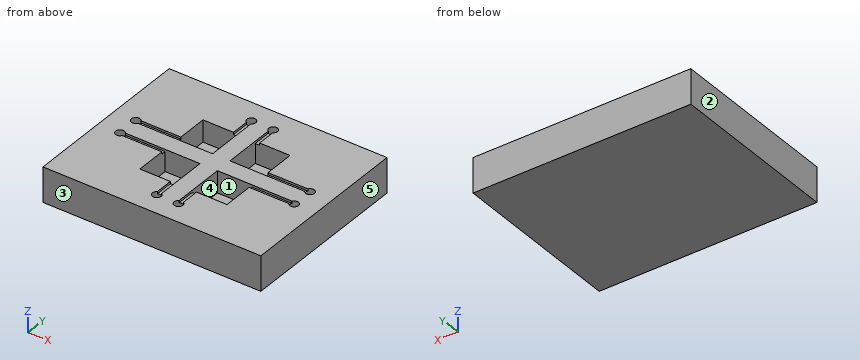
from build123d import *

# Parameters (mm, degrees)
F0_W     = 8
F0_H     = 8
F1_DEPTH = 5
F2_W     = 50
F2_H     = 40
F3_DEPTH = 3
F4_W     = 1
F4_H     = 5
F4_W_2   = 10
F4_H_2   = 1
F5_DEPTH = 0.5
F6_R     = 1
F7_DEPTH = 5


with BuildPart() as f1:
    # F0 (on Top) → F1 (new body)
    with BuildSketch(Plane.XY):
        Polygon((-25, -20), (25, -20), (25, 20), (-10, 20), (-25, 20), align=None)
        with Locations((-6, -6)):
            Rectangle(F0_W, F0_H, mode=Mode.SUBTRACT)
        with Locations((6, -6)):
            Rectangle(F0_W, F0_H, mode=Mode.SUBTRACT)
        with Locations((-6, 6)):
            Rectangle(F0_W, F0_H, mode=Mode.SUBTRACT)
        with Locations((6, 6)):
            Rectangle(F0_W, F0_H, mode=Mode.SUBTRACT)
    extrude(amount=F1_DEPTH)

    # F2 (on face) → F3 (join)
    with BuildSketch(Plane(origin=(0, 0, 0), x_dir=(1, 0, 0), z_dir=(0, 0, -1))):
        Rectangle(F2_W, F2_H)
    extrude(amount=F3_DEPTH)

    # F4 (on face) → F5 (cut)
    with BuildSketch(Plane.XY.offset(5)):
        with Locations((2.5, -12.5)):
            Rectangle(F4_W, F4_H)
        with Locations((-2.5, -12.5)):
            Rectangle(F4_W, F4_H)
        with Locations((-2.5, 12.5)):
            Rectangle(F4_W, F4_H)
        with Locations((2.5, 12.5)):
            Rectangle(F4_W, F4_H)
        with Locations((15, -2.5)):
            Rectangle(F4_W_2, F4_H_2)
        with Locations((15, 2.5)):
            Rectangle(F4_W_2, F4_H_2)
        with Locations((-15, 2.5)):
            Rectangle(F4_W_2, F4_H_2)
        with Locations((-15, -2.5)):
            Rectangle(F4_W_2, F4_H_2)
    extrude(amount=-F5_DEPTH, mode=Mode.SUBTRACT)

    # F6 (on face) → F7 (cut)
    with BuildSketch(Plane.XY.offset(5)):
        with Locations((20, -2.5)):
            Circle(F6_R)
        with Locations((20, 2.5)):
            Circle(F6_R)
        with Locations((-20, -2.5)):
            Circle(F6_R)
        with Locations((-20, 2.5)):
            Circle(F6_R)
        with Locations((2.5, -15)):
            Circle(F6_R)
        with Locations((-2.5, -15)):
            Circle(F6_R)
        with Locations((2.5, 15)):
            Circle(F6_R)
        with Locations((-2.5, 15)):
            Circle(F6_R)
    extrude(amount=-F7_DEPTH, mode=Mode.SUBTRACT)


solid = f1.part
Work out the finished part from the listing and answer in its coordinate system (mm). Face numbers are marked on the shaded views. A direction names the side the tool comes from. Round coordinates to 2 decimals unless told otherwise and drop trailing zeros. Loops run counter-clockwise (first coordinate to the right, second up) from the corner with the lowest first, then second, coordinate; pieces in that order, holes last. Notation, with made-up numbers: (36, 74) - (83, 74) arc R13 cw to (83, 95) - close; hole circle Ø7 at (84.5, 41). An arc over 180 degrees is marked (long way). One line per item, written item: value.
Q1. Straight lines are drawn through the part: probe 1 along Y at (x, z) = (2.5, 3.5); probe 2 along Y at (x, z) = (-20, 1.45); probe 3 along X at (y, z) = (2.5, 3.85). For each, find the intervals that lie inside material, in ascending order.
Check values:
probe 1: -20 to -16, -14 to -10, -2 to 2, 10 to 14, 16 to 20
probe 2: -20 to -3.5, -1.5 to 1.5, 3.5 to 20
probe 3: -25 to -21, -19 to -10, -2 to 2, 10 to 19, 21 to 25
Q2. Each of these flat-tipped pins is pushed along its axis until it touches: pin 1 Ø9 at (x, y) = (5.5, -5.5) entering from +Z; pin 2 Ø0.8 at (x, y) = (-2.5, 12.5) entering from +Z; pin 3 Ø4 at (x, y) = (-6, 5.5) entering from +Z. Where does it stop, or does it pass through?
Check values:
pin 1: z = 5
pin 2: z = 4.5
pin 3: z = 0
Q3. Find section B-B on z = 3.5. State how many separate pieces and enclosed holes the cut face has, and give its area (3 significant figures).
Check values:
separate pieces: 1
enclosed holes: 12
area: 1,720 mm2
Q4. For the marked faces 1 and 2, determine the directions among +Z, -Z, +X, -X, +Y, -Y from which every point of the face is accessible in a straight line to the end or side of a thin tool.
Check values:
face 1: +Z
face 2: +Z, -Z, -X, +Y, -Y
Q5. The mould has two halves that part along X. Classify the marked faces 3, 4 and 5: +X half, -X half, draft (parallel to the pull), parting line (faces both ways), or undercut.
Check values:
face 3: draft
face 4: undercut
face 5: +X half
Q6. Find section A-A on x = 6. Give the vertices of the cut face in (y, z), and give its area (3 significant figures).
Check values:
outline: (-20, -3) - (20, -3) - (20, 5) - (10, 5) - (10, 0) - (2, 0) - (2, 5) - (-2, 5) - (-2, 0) - (-10, 0) - (-10, 5) - (-20, 5) - close
area: 240 mm2
Q7. Find section C-C on y = 8.5. Give the vertices of the cut face in (x, z).
Check values:
outline: (-25, -3) - (25, -3) - (25, 5) - (10, 5) - (10, 0) - (2, 0) - (2, 5) - (-2, 5) - (-2, 0) - (-10, 0) - (-10, 5) - (-25, 5) - close
